Design review of the part built by this model. Coordinates are the model's own, in mm. Face numbers are marked on the shaded views. A direction names the side the tool comes from. Give positions to 0.01 mm unless a question says otherwise; leave off trailing zeros. Loops run counter-clockwise (first coordinate to the right, second up) from the corner with the lowest first, then second, coordinate; pieces in that order, holes last. Notation, with made-up numbers: M 54,-24 L 98,-24 A14 ccw 98,-5 Z; hole C 84,31 d2. An arc over 180 degrees is marked long. Use one line per item in the form item = value. Start each with the question number.
Autodesk Inventor part; units mm, degrees
ref_plane "Work Plane1" through (29, 0, 0) normal (0, -1, 0) x (1, 0, 0)
ref_plane "YZ Plane" through (0, 0, 0) normal (1, 0, 0) x (0, 1, 0)
ref_plane "XZ Plane" through (0, 0, 0) normal (0, 1, 0) x (-1, 0, 0)
sketch "Rascunho1" plane through (0, 0, 0) normal (0, 0, 1) x (1, 0, 0)
  line L0 (-2.6667, 0) -> (65, 0)
  line L1 (65, 0) -> (65, 6)
  line L2 (65, 6) -> (29, 6)
  line L3 (29, 6) -> (27.9264, 6)
  line L4 (27.9264, 6) -> (0, 6)
  line L5 (0, 6) -> (0, 9)
  line L6 (0, 9) -> (-12, 9)
  line L7 (-12, 9) -> (-12, 5.7735)
  line L8 (-12, 5.7735) -> (-6, 5.7735)
  line L9 (-6, 5.7735) -> (-2.6667, 0)
  line L10 (-34.4, 0) -> (122.4, 0)
  line L11 (0, -1.8) -> (0, 10.8)
  line L12 (29, 6) -> (0, 6) construction
  dimension "d1" = 36
  dimension "d2" = 1.0736
  dimension "d3" = 12
  dimension "d4" = 6
  dimension "d5" = 60
  dimension "d6" = 12
  dimension "d7" = 12
  dimension "d8" = 11.547
  dimension "d9" = 18
  dimension "d26" = 65
revolve "Corpo" add sketch "Rascunho1" angle 360 about axis through (-2.6667, 0, 0) along (1, 0, 0)
sketch "Rascunho2" plane through (-12, 0, 0) normal (-1, 0, 0) x (0, 0, 1)
  circle A0 centre (0, 0) radius 5.7735
  line L0 (0, -12.6) -> (0, 12.6)
  line L1 (-12.6, 0) -> (12.6, 0)
  line L2 (5.7735, 0) -> (2.8868, -5)
  line L3 (2.8868, -5) -> (-2.8868, -5)
  line L4 (-2.8868, -5) -> (-5.7735, 0)
  line L5 (-5.7735, 0) -> (-2.8868, 5)
  line L6 (-2.8868, 5) -> (2.8868, 5)
  line L7 (2.8868, 5) -> (5.7735, 0)
extrude "Fenda" add sketch "Rascunho2" against normal up to next contours L7 A0 | A0 L2 | L6 L0 A0 | A0 L0 L3 | L0 L6 A0 | A0 L3 L0 | L4 A0 | A0 L5
fillet "Raio de arredondamento1" radius 1.2 1 edges at (-12, -9, 0)
thread "Rosca"
chamfer "Chanfrar1" distance 1.0735 distance2 1.0735 1 edges at (65, -6, 0) measured on face at (65, -1.5551, 1.8049)
ref_plane "Work Plane1" through (29, 0, 0) normal (0, -1, 0) x (1, 0, 0)
fillet "Fillet2" radius 0.1 1 edges at (0, -6, 0)
equation "\"d1\" = GEL"
equation "\"d3\" = KOH"
equation "\"d4\" = INTI"
equation "\"d6\" = GD"
equation "\"d7\" = BDM"
equation "\"d8\" = 1.1547 * SW"
equation "\"d9\" = KOD"
equation "\"d26\" = NLG"
equation "\"d17\" = RR"
equation "\"d13\" = GEL"
equation "\"d15\" = -0.5 * SPD + 0.5 * GD"
equation "\"d16\" = GUL"
equation "\"d30\" = R"
equation "\"GD\" = NND"
equation "\"NLG\" = 65"
equation "\"GEL\" = 36"
equation "\"KOD\" = 18"
equation "\"KOH\" = 12"
equation "\"INTI\" = 6"
equation "\"GAL\" = 0.61345 * PTC"
equation "\"GUL\" = 0.61345 * PTC"
equation "\"BDM\" = NND"
equation "\"RR\" = 1.2"
equation "\"SPD\" = NND - 1.2269 * PTC"
equation "\"R\" = 0.1"
equation "\"TOA\" = 30deg"
equation "\"GD1\" = THREADDIA - 1.2269 * PTC"
equation "\"THREADDIA\" = 12"
equation "\"FAWI\" = 45deg"
equation "\"ANG\" = 120deg"
equation "\"PTC\" = 1.75"
equation "\"NND\" = 12"
equation "\"E0\" = 1.155 * SW"
properties part number "DIN 912 - M12x65" material "Aço Inox AISI 304"
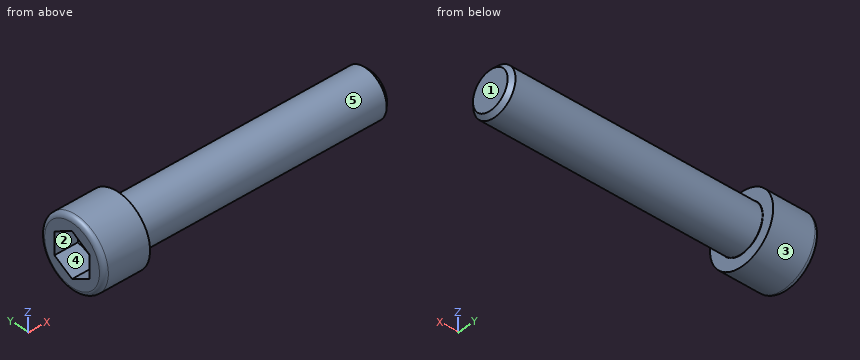
Q1. The part is to be moulded in two halves that separate along Z. For the marked faces 1, 2 and 3, say which applies: pulls with the +Z half, pulls with the -Z half, needs draft (parallel to the pull), parting line crosses it, or undercut.
Q2. Take a section at A-A on x = 25.5. Give the boundary of the cut face in (y, z).
Q3. Wall thickness on probe 1 along X at (y, z) = (3.25, -5.5); probe 2 along Z at (x, y) = (42.5, 0); probe 3 along X at (y, z) = (-0.5, -1): over which ranges is each line inside the solid? List them lowest first.
Q4. For the marked faces 4 and 5, list the 3-axis set-ups (+Z, -Z, +X, -X, +Y, -Y) from which the entire face can be reached by the end or side of a thin tool; tool diameter is ignored.
Q5. Clearance check with flat-ended pins moving along their axes: pin 1 Ø1 at (x, z) = (25.5, -2.5) entering from +Y; pin 2 Ø1.5 at (y, z) = (-5.5, 5) entering from +X; pin 3 Ø10 at (x, z) = (26, -1) entering from +Y. State where each tip first meets the part, or that it passes through.
Response values:
q1.face_1 = needs draft
q1.face_2 = undercut
q1.face_3 = parting line crosses it
q2.outline = C 0,0 d12
q3.probe_1 = -12 to 0
q3.probe_2 = -6 to 6
q3.probe_3 = -3.31 to 65
q4.face_4 = -X
q4.face_5 = +X
q5.pin_1 = 5.66
q5.pin_2 = 0
q5.pin_3 = 6
